Build history of the part. All positions in model axes, mm. Face numbers are marked on the shaded views. Round coordinates to 2 decimals unless told otherwise and drop trailing zeros. Write each loop counter-clockwise with the first axis right and the second up, starting at its lowest first coordinate (ties: lowest second). Pieces come first, ordered by that corner, then holes. Notation, with made-up numbers: (2.25, 45.5) -> (46.25, 45.5) arc R10 cw to (46.25, 61.5) -> close; hole circle Ø8 at (-29.75, 12.5). An arc over 180 degrees is marked (long way). One line per question, with ' | ' between items.
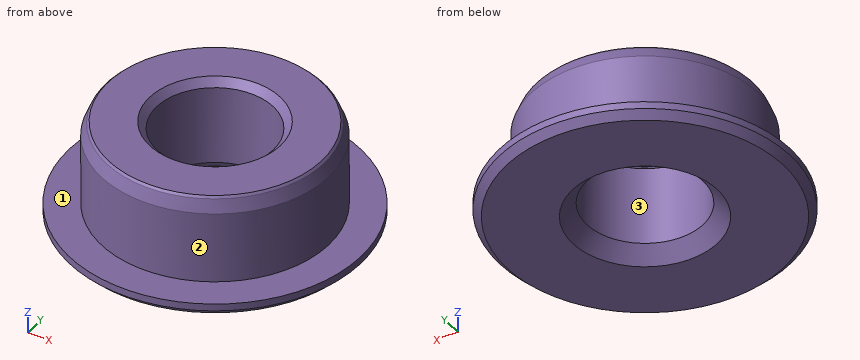
from build123d import *

# Parameters (mm, degrees)
F0_R     = 10.25
F0_R_2   = 8
F1_DEPTH = 1
F0_R_3   = 4.105
F2_DEPTH = 7
F3_SIZE  = 0.5
F4_SIZE  = 0.5
F5_SIZE  = 0.5
F6_SIZE  = 1


with BuildPart() as f1:
    # F0 (on Top) → F1 (new body)
    with BuildSketch(Plane.XY):
        Circle(F0_R)
        Circle(F0_R_2, mode=Mode.SUBTRACT)
    extrude(amount=F1_DEPTH)

    # F0 (on Top) → F2 (join)
    with BuildSketch(Plane.XY):
        Circle(F0_R_2)
        Circle(F0_R_3, mode=Mode.SUBTRACT)
    extrude(amount=F2_DEPTH)

    # F3
    f3_edges = [f1.edges().sort_by_distance(p)[0] for p in [
        (-10.25, 0, 0),
        (-4.105, 0, 7),
    ]]
    chamfer(f3_edges, length=F3_SIZE)

    # F4
    f4_edges = [f1.edges().sort_by_distance(p)[0] for p in [
        (-8, 0, 7),
    ]]
    chamfer(f4_edges, length=F4_SIZE)

    # F5
    f5_edges = [f1.edges().sort_by_distance(p)[0] for p in [
        (-8, 0, 6.5),
    ]]
    chamfer(f5_edges, length=F5_SIZE)

    # F6
    f6_edges = [f1.edges().sort_by_distance(p)[0] for p in [
        (-4.105, 0, 0),
    ]]
    chamfer(f6_edges, length=F6_SIZE)


solid = f1.part
(1) Mould opens along X. For the marked faces 1, 2 and 3 say: pulls with the +X half, pulls with the -X half, needs draft (parallel to the pull), parting line crosses it, or undercut.
Calculated:
face 1: needs draft | face 2: parting line crosses it | face 3: undercut
(2) Wall check: line 1 (Y direction, x = 0, z = 2.35) (3 decimals); line 2 (Z direction, x = -8.5, y = 4.75); line 3 (Y direction, x = -3, z = 3.25). Give the ranges that are in metal, low to high. Write a range as from..to.
Calculated:
line 1: -8..-4.105, 4.105..8 | line 2: 0..1 | line 3: -7.42..-2.8, 2.8..7.42
(3) Slice it at A-A (z = 3). Write the cut outline in (x, y) (3 decimals), then the cut area to 3 significant figures.
Calculated:
outline: circle Ø16 at (0, 0); hole circle Ø8.21 at (0, 0) | area: 148 mm2
(4) Drop flat-ended pins along their axis: pin 1 (4 mm diameter, centred on y = 5.5, z = 1, fed in from +X); pin 2 (9.5 mm diameter, centred on x = 0, y = 0, fed in from -Z) (3 decimals); pin 3 (3 mm diameter, centred on y = -2.5, z = 6, fed in from +X); pin 4 (1.5 mm diameter, centred on x = 2, y = -0.5, fed in from -Z). Give the stop position or say it passes through.
Calculated:
pin 1: x = 9.63 | pin 2: z = 0.355 | pin 3: x = 7.94 | pin 4: through
